from build123d import *

# Parameters (mm, degrees)
F0_W          = 20
F0_H          = 10.77
F1_DEPTH      = 10
F1_DEPTH_BACK = 20
F3_DEPTH      = 30
F3_DEPTH_BACK = 10
F4_DEPTH      = 10
F5_R          = 1.15
F6_DEPTH      = 25
F7_W          = 9
F7_H          = 5.77
F8_DEPTH      = 15
F9_R          = 2.5
F10_R         = 2.5


with BuildPart() as f1:
    # F0 (on Top) → F1 (new body, two sides)
    with BuildSketch(Plane.XY) as f1_sk:
        with Locations((4.4768884756, -0.816908665)):
            Rectangle(F0_W, F0_H)
    extrude(amount=F1_DEPTH)
    extrude(f1_sk.sketch, amount=-F1_DEPTH_BACK)

    # F2 (on face) → F3 (join, two sides)
    with BuildSketch(Plane(origin=(-5.5231115244, 0, 0), x_dir=(0, -1, 0), z_dir=(-1, 0, 0))) as f3_sk:
        Polygon((7.9035344876, 42.4689549124), (8.6624058531, 56.9490831664), (4.6678877141, 57.1584269913), (3.2377782985, 29.8703137532), (-4.568091335, 22.4698111415), (-4.568091335, 10), (6.201908665, 10), (7.4136699372, 33.1217824671), align=None)
    extrude(amount=-F3_DEPTH)
    extrude(f3_sk.sketch, amount=F3_DEPTH_BACK)

    # F4 (add): a face of the model
    f4_faces = [f1.faces().sort_by_distance(p)[0] for p in [
        (4.4768884756, -6.6651467836, 57.0537550789),
    ]]
    extrude(f4_faces, amount=F4_DEPTH)

    # F5 (on face) → F6 (cut)
    with BuildSketch(Plane(origin=(0, -5.6622789964, -0.2967474679), x_dir=(1, 0, 0), z_dir=(0, -0.9986295348, -0.0523359562))):
        Polygon((8.7768884756, 48.1932846266), (4.4768884756, 48.1932846266), (0.1768884756, 48.1932846266), (0.1768884756, 39.5932846266), (8.7768884756, 39.5932846266), align=None)
        with Locations((14.9768884756, 56.4432846266)):
            Circle(F5_R)
        with Locations((14.9768884756, 44.0432846266)):
            Circle(F5_R)
        with Locations((-6.0231115244, 44.0432846266)):
            Circle(F5_R)
        with Locations((-6.0231115244, 56.4432846266)):
            Circle(F5_R)
    extrude(amount=-F6_DEPTH, mode=Mode.SUBTRACT)

    # F7 (on face) → F8 (join)
    with BuildSketch(Plane(origin=(0, 0, -20), x_dir=(1, 0, 0), z_dir=(0, 0, -1))):
        with Locations((4.4768884756, 0.816908665)):
            Rectangle(F7_W, F7_H)
    extrude(amount=F8_DEPTH)

    # F9
    f9_edges = [f1.edges().sort_by_distance(p)[0] for p in [
        (-15.523112, -7.188506, 67.04005),
        (24.476888, -7.188506, 67.04005),
    ]]
    fillet(f9_edges, radius=F9_R)

    # F10
    f10_edges = [f1.edges().sort_by_distance(p)[0] for p in [
        (4.476888, -3.237778, 29.870314),
        (4.476888, 4.568091, 22.469811),
    ]]
    fillet(f10_edges, radius=F10_R)


solid = f1.part
Model file for the job. Use its own axes, mm. A direction names the side the tool comes from. Give positions to 0.01 mm unless a question says otherwise; leave off trailing zeros. Write each loop counter-clockwise with the first axis right and the second up, starting at its lowest first coordinate (ties: lowest second). Pieces come first, ordered by that corner, then holes. Notation, with made-up numbers: (-19.5, 59.5) - (-0.5, 59.5) arc R23 cw to (-0.5, 81.5) - close; hole circle Ø3 at (24, 5.25). An arc over 180 degrees is marked (long way). Answer as CSV lines item,"result".
1. 3-axis set-ups, long thin cutter, end or side, ignore diameter. For faces 1 (the face through (-5.523, -1, -5)), 2 (the face through (4, -3.702, -27)), 3 (the face through (4, 2.068, -27)): which of +Z, -Z, +X, -X, +Y, -Y reach the whole face in a straight line?
Responses:
face 1,"-Z, -X, +Y, -Y"
face 2,"-Z, +X, -X, -Y"
face 3,"-Z, +X, -X, +Y"
2. Band-saw the part on B-B (x = 17.5). Write the cut outline in (y, z), and give its area (3 significant figures).
Responses:
outline,"(-9.19, 66.94) - (-6.2, 10) - (4.57, 10) - (4.57, 21.4) arc R2.5 ccw to (3.79, 23.21) - (-2.51, 29.18) arc R2.5 cw to (-3.29, 30.87) - (-5.19, 67.14) - close"
area,"344 mm2"
3. Two-plate mould, pull along Z, no slides. Class faces 4 (the face through (4.72, -7.22, 67.04)), 5 (the face through (14.477, -1, -5)), 6 (the face through (4.537, -6.215, 47.934)): +Z half, -Z half, draft (parallel to the pull), parting line (faces both ways), or undercut.
Responses:
face 4,"+Z half"
face 5,"draft"
face 6,"undercut"
4. Band-saw the part on D-D (z = 0.5). Write the cut outline in (x, y).
Responses:
outline,"(-5.52, -6.2) - (14.48, -6.2) - (14.48, 4.57) - (-5.52, 4.57) - close"
5. Band-saw the part on C-C (y = 0.5). Write the cut outline in (x, z), and give its area (3 significant figures).
Responses:
outline,"(-15.52, 10) - (-5.52, 10) - (-5.52, -20) - (-0.02, -20) - (-0.02, -35) - (8.98, -35) - (8.98, -20) - (14.48, -20) - (14.48, 10) - (24.48, 10) - (24.48, 26.33) - (-15.52, 26.33) - close"
area,"1,390 mm2"
6. Band-saw the part on A-A (x = 4). Write the cut outline in (y, z).
Responses:
outline,"(-9.19, 66.94) - (-8.18, 47.83) - (-4.19, 48.04) - (-5.19, 67.14) - close; (-7.73, 39.24) - (-6.2, 10) - (-6.2, -20) - (-3.7, -20) - (-3.7, -35) - (2.07, -35) - (2.07, -20) - (4.57, -20) - (4.57, 21.4) arc R2.5 ccw to (3.79, 23.21) - (-2.51, 29.18) arc R2.5 cw to (-3.29, 30.87) - (-3.74, 39.45) - close"
7. Drill centre lines: L1, parallel to X at y = -7, z = 40.5; L2, parallel to X at y = 2.75, z = -2.5; L3, parallel to Z at x = 2.5, y = -4. Where is each one in solid material? Low to high. Write a range as [from, to].
Responses:
L1,"x = [-15.52, 0.18], [8.78, 24.48]"
L2,"x = [-5.52, 14.48]"
L3,"z = [-20, 39.44]"
8. Pin check, flat tips, straight feed: pin 1 (16 mm diameter, centred on x = 7, z = -8.5, fed in from -Y); pin 2 (5.5 mm diameter, centred on y = -3, z = 1.5, fed in from -X); pin 3 (3 mm diameter, centred on x = -9, y = 0.5, fed in from +Z); pin 4 (2 mm diameter, centred on x = -8, z = 4, fed in from -Y). Stop position of each tip, or through.
Responses:
pin 1,"stops at y = -6.2"
pin 2,"stops at x = -5.52"
pin 3,"stops at z = 27.75"
pin 4,"passes through"
